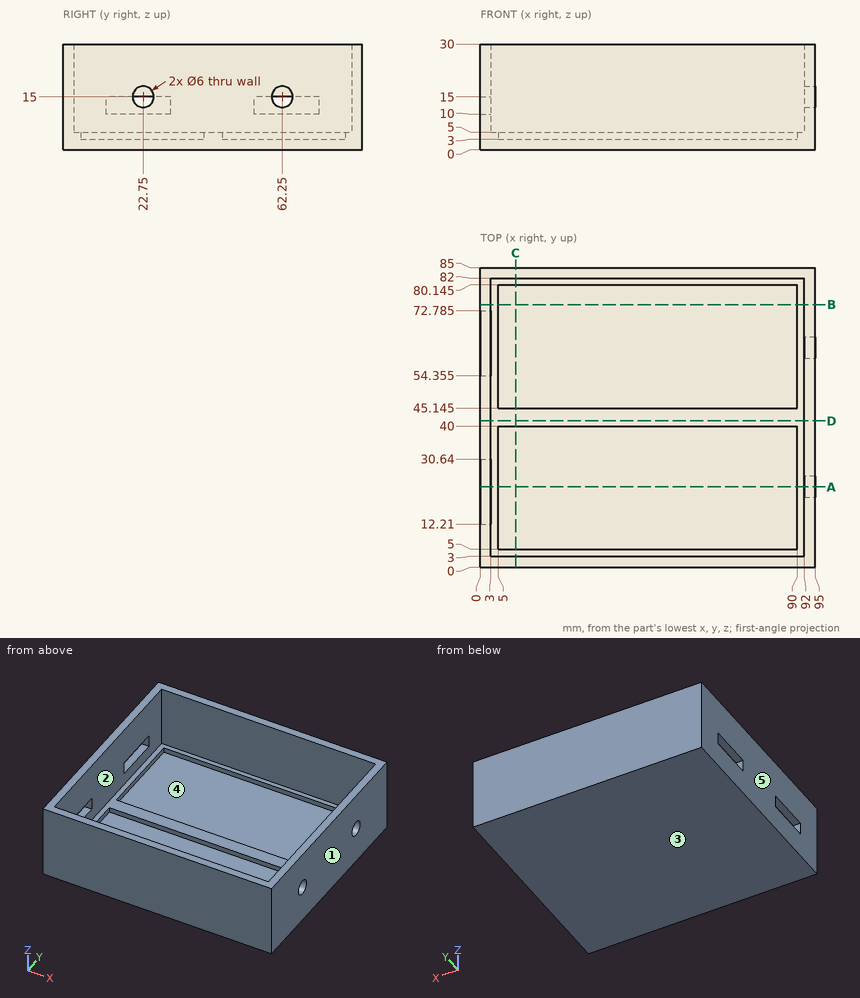
Input: dimensioned drawing with shaded views. Units: mm. Origin: part minimum x, y, z. A direction names the side the tool comes from. Give positions to 0.01 mm unless a question says otherwise; leave off trailing zeros. Write each loop counter-clockwise with the first axis right and the second up, starting at its lowest first coordinate (ties: lowest second). Pieces come first, ordered by that corner, then holes. Notation, with made-up numbers: M -30,32.25 L 15,32.25 A17 ccw 15,40.25 Z; hole C 65.25,-17 d6. An arc over 180 degrees is marked long. Return JSON: item names as keys, results as strings. Group by question number.
1) Cut plane D-D, the plane y = 41.5. Output: boundary loops of the cut face in (x, z).
2) Pull-direction query (X, two-part tool) for the marked faces 3, 4 and 5; classes: pulls with the +X half, pulls with the -X half, needs draft (parallel to the pull), parting line crosses it, or undercut.
3) Pin query (flat end, axial travel): P1, Ø8, axis at x = 60, y = 10.5, coming from the +Z side; P2, Ø23.5, axis at x = 68, y = 34.5, coming from the +Z side. Return the tip coordinate at first contact, or that it passes through.
4) Material intervals for line 1 along X through (y, z) = (15, 18.25); line 2 along X through (y, z) = (64, 3.25); line 3 along Y through (x, z) = (76, 5.75), sorted ascending. Write a range as [from, to].
5) Cut plane A-A, the plane y = 22.75. Output: boundary loops of the cut face in (x, z).
6) Cut plane C-C, the plane x = 10. Output: boundary loops of the cut face in (y, z) (3 decimals).
7) Set-up query: the marked faces 1 and 2. Return all of +Z, -Z, +X, -X, +Y, -Y with unobstructed straight access to the full face (end or side cutting, diameter ignored); none if empty.
8) Cut plane B-B, the plane y = 74.5. Output: boundary loops of the cut face in (x, z), plus the area to 3 significant figures.
Recorded:
{
 "1": {"outline": "M 0,0 L 95,0 L 95,30 L 92,30 L 92,5 L 3,5 L 3,30 L 0,30 Z"},
 "2": {"face 3": "needs draft", "face 4": "undercut", "face 5": "pulls with the -X half"},
 "3": {"P1": "stops at z = 3", "P2": "stops at z = 5"},
 "4": {"line 1": "x = [0, 3], [92, 95]", "line 2": "x = [0, 5], [90, 95]", "line 3": "y = [0, 3], [82, 85]"},
 "5": {"outline": "M 0,0 L 95,0 L 95,12 L 92,12 L 92,5 L 90,5 L 90,3 L 5,3 L 5,5 L 3,5 L 3,10 L 0,10 Z; M 0,15 L 3,15 L 3,30 L 0,30 Z; M 92,18 L 95,18 L 95,30 L 92,30 Z"},
 "6": {"outline": "M 0,0 L 85,0 L 85,30 L 82,30 L 82,5 L 80.145,5 L 80.145,3 L 45.145,3 L 45.145,5 L 40,5 L 40,3 L 5,3 L 5,5 L 3,5 L 3,30 L 0,30 Z"},
 "7": {"face 1": "+Z, -Z, +X, +Y, -Y", "face 2": "+Z"},
 "8": {"outline": "M 0,0 L 95,0 L 95,30 L 92,30 L 92,5 L 90,5 L 90,3 L 5,3 L 5,5 L 3,5 L 3,30 L 0,30 Z", "area": "455 mm²"}
}
